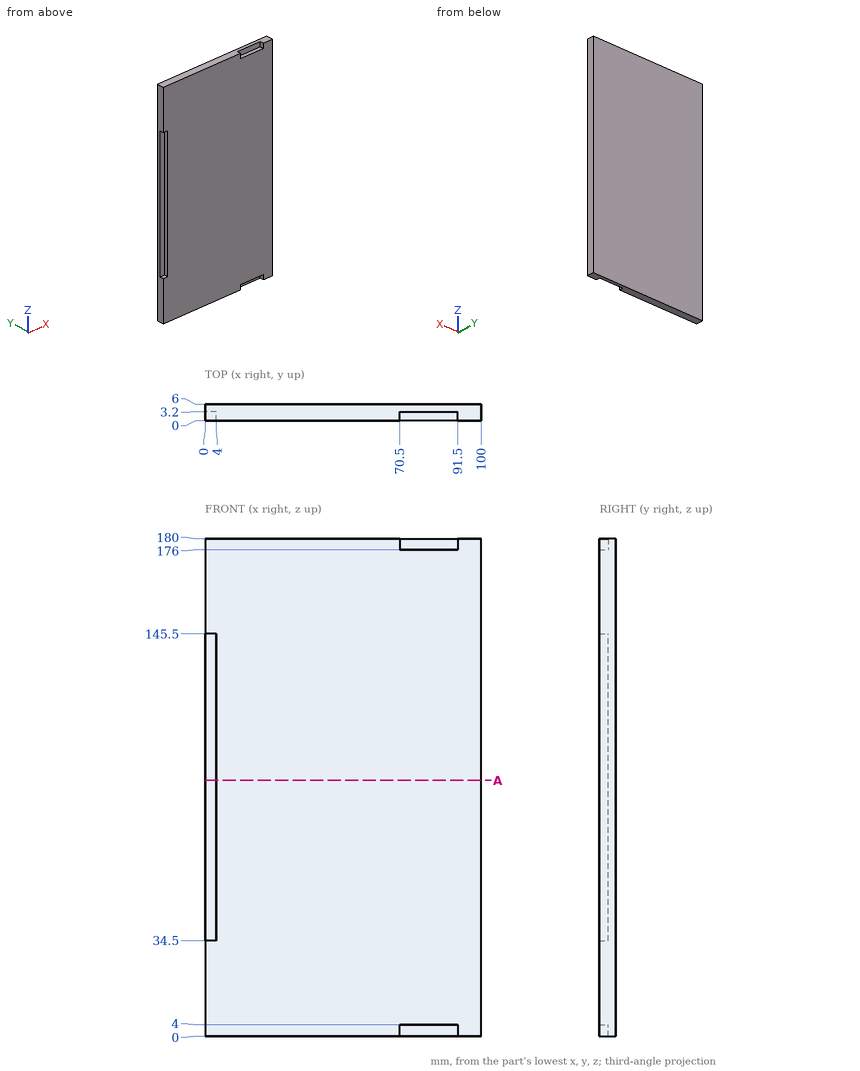
Study the drawing (mm; zero at the part's minimum x, y, z) and answer. Round coordinates to 2 decimals unless told otherwise and drop trailing zeros. Loops run counter-clockwise (first coordinate to the right, second up) from the corner with the lowest first, then second, coordinate; pieces in that order, holes last.
Q1. Find the intervals of material crossed by line 1 (X direction, y = 2.4, z = 125); line 2 (Z direction, x = 90, y = 2.2), in increasing order.
Q2. Section A-A, the plane z = 92.5 is taken. Determine the outline of the cut face in (x, y).
Q3. Given pin 1 Ø2.5 at (x, y) = (76.5, 1) entering from +Z; pin 2 Ø1 at (x, y) = (79, 2.5) entering from -Z; pin 3 Ø2 at (x, z) = (85, 2.5) entering from -Y, each flat-ended and moving along its own axis, determine where each tip first touches the part or whether it passes through.
Completed:
1. line 1: x = 4 to 100
1. line 2: z = 4 to 176
2. outline: (0, 3.2) - (4, 3.2) - (4, 0) - (100, 0) - (100, 6) - (0, 6) - close
3. pin 1: stops at z = 176
3. pin 2: stops at z = 4
3. pin 3: stops at y = 3.2
